Autodesk Inventor part; units mm, degrees
ref_plane "YZ Plane" through (0, 0, 0) normal (1, 0, 0) x (0, 1, 0)
ref_plane "XZ Plane" through (0, 0, 0) normal (0, 1, 0) x (-1, 0, 0)
ref_plane "XY Plane" through (0, 0, 0) normal (0, 0, 1) x (1, 0, 0)
sketch "Sketch1" plane through (0, 0, 0) normal (0, 0, 1) x (1, 0, 0)
  circle A0 centre (0, 0) radius 3.3
  dimension "d0" = 6.6
extrude "Extrusion1" add sketch "Sketch1" along normal blind 2.7
fillet "Fillet1" radius 2 1 edges at (-3.3, 0, 2.7)
sketch "Sketch2" plane through (0, 0, 0) normal (0, 0, -1) x (-1, 0, 0)
  circle A0 centre (0, 0) radius 2
  dimension "d4" = 4
extrude "Extrusion2" add sketch "Sketch2" along normal blind 4
thread "Thread1"
properties part number "round m4x5"
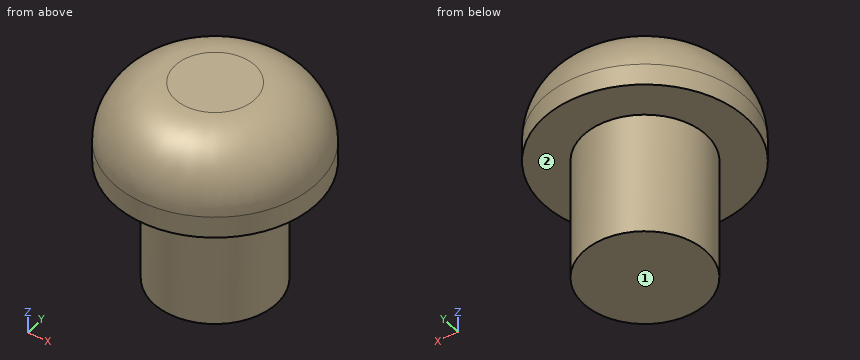
Work out the finished part from the listing and answer in its coordinate system (mm). Face numbers are marked on the shaded views. A direction names the side the tool comes from. Give positions to 0.01 mm unless a question says otherwise; leave off trailing zeros. Loops run counter-clockwise (first coordinate to the right, second up) from the corner with the lowest first, then second, coordinate; pieces in that order, holes last. Notation, with made-up numbers: (3.25, 31) -> (30.25, 31) arc R25 ccw to (30.25, 54) -> close; hole circle Ø2 at (1.5, 61). An arc over 180 degrees is marked (long way). One line per question, with ' | ' between items. Start each with the question number.
1) For the marked faces 1 and 2, determine the directions among +Z, -Z, +X, -X, +Y, -Y from which every point of the face is accessible in a straight line to the end or side of a thin tool.
2) Straight lines are drawn through the part: L1, parallel to X at y = 2.5, z = 2; L2, parallel to Y at x = 2, z = 2; L3, parallel to X at y = 1.5, z = 1.75. For each, find the intervals that lie inside material, in ascending order.
3) Section A-A, the plane z = 0.25 is taken. Determine the outline of the cut face in (x, y).
Resolved:
1) face 1: -Z, +X, -X, +Y, -Y | face 2: -Z
2) L1: -1.3 to 1.3 | L2: -1.99 to 1.99 | L3: -2.6 to 2.6
3) outline: circle Ø6.6 at (0, 0)
